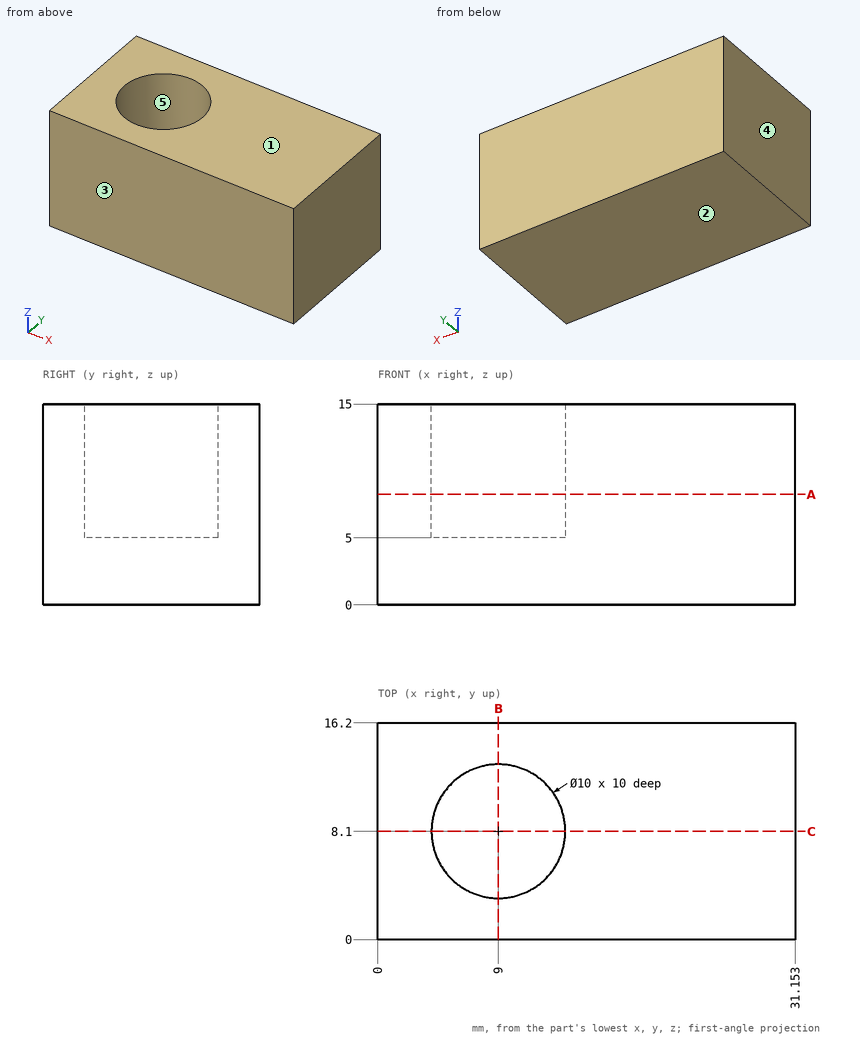
Answer from the drawing. Dimensions are ordinates in mm from the lowest x, y and z of the part. A direction names the side the tool comes from. Give positions to 0.01 mm unless a question says otherwise; leave off trailing zeros. Write each loop counter-clockwise with the first axis right and the second up, starting at its lowest first coordinate (ties: lowest second). Pieces come first, ordered by that corner, then holes. Notation, with made-up numbers: (9.5, 54) - (27.5, 54) arc R13 cw to (27.5, 70) - close; hole circle Ø7 at (-12, -39). An arc over 180 degrees is marked (long way). One line per item, written item: value. Start each with the question number.
1. Find section B-B (x = 9). Write down the section's boundary in (y, z).
2. For the marked faces 4 and 5, determine the directions among +Z, -Z, +X, -X, +Y, -Y from which every point of the face is accessible in a straight line to the end or side of a thin tool.
3. Consider probe 1 along Y at (x, z) = (9, 11); probe 2 along Z at (x, y) = (5.5, 7.25); probe 3 along X at (y, z) = (7.75, 9.75). Determine where each line is inside the solid, lowest interval first.
4. Given pin 1 (3 mm diameter, centred on x = 11, z = 5.5, fed in from -Y), flat-ended and moving along its own axis, determine where the tip first touches the part or whether it passes through.
5. For a pull along Z with two mould halves and no side action, classify the marked faces 1, 2 and 3 as +Z half, -Z half, draft (parallel to the pull), parting line (faces both ways), or undercut.
6. Find section C-C (y = 8.1). Write down the section's boundary in (x, z).
7. Find section A-A (z = 8.25). Write down the section's boundary in (x, y), then the cut area to 3 significant figures.
Geometry results:
1. outline: (0, 0) - (16.2, 0) - (16.2, 15) - (13.1, 15) - (13.1, 5) - (3.1, 5) - (3.1, 15) - (0, 15) - close
2. face 4: +Z, -Z, -X, +Y, -Y
2. face 5: +Z
3. probe 1: 0 to 3.1, 13.1 to 16.2
3. probe 2: 0 to 5
3. probe 3: 0 to 4.01, 13.99 to 31.15
4. pin 1: y = 0
5. face 1: +Z half
5. face 2: -Z half
5. face 3: draft
6. outline: (0, 0) - (31.15, 0) - (31.15, 15) - (14, 15) - (14, 5) - (4, 5) - (4, 15) - (0, 15) - close
7. outline: (0, 0) - (31.15, 0) - (31.15, 16.2) - (0, 16.2) - close; hole circle Ø10 at (9, 8.1)
7. area: 426 mm2
